from build123d import *

# Parameters (mm, degrees)
SKETCH1_R           = 12.5
BOSS_EXTRUDE1_DEPTH = 75
SKETCH2_R           = 15
BOSS_EXTRUDE2_DEPTH = 20
FILLET1_R           = 2


# Read off the part's stored shape, not the designer's step: Shell2
with BuildPart() as part:
    # Sketch1 → Boss-Extrude1 (new, symmetric)
    with BuildSketch(Plane(origin=(0, 0, 0), x_dir=(1, 0, 0), z_dir=(0, 1, 0))):
        with Locations(Location((0, 0, 0), (0, 0, 270))):
            Circle(SKETCH1_R)
    extrude(amount=BOSS_EXTRUDE1_DEPTH, both=True)

    # Sketch2 → Boss-Extrude2 (add)
    with BuildSketch(Plane(origin=(0, 75, 0), x_dir=(1, 0, 0), z_dir=(0, 1, 0))):
        with Locations(Location((0, 0, 0), (0, 0, 270))):
            Circle(SKETCH2_R)
    boss_extrude2 = extrude(amount=-BOSS_EXTRUDE2_DEPTH)

    # Mirror1: Boss-Extrude2 across plane
    add(boss_extrude2.mirror(Plane.ZX))

    # Fillet1
    fillet1_edges = [part.edges().sort_by_distance(p)[0] for p in [
        (0, -75, -15),
        (0, 75, -15),
    ]]
    fillet(fillet1_edges, radius=FILLET1_R)

    # Shell2 outline → Shell2 (revolve, cut)
    with BuildSketch(Plane.XY):
        with BuildLine():
            Line((13, 74), (0, 74))
            Line((0, 74), (0, -74))
            Line((0, -74), (13, -74))
            ThreePointArc((13, -74), (13.707106781, -73.707106781), (14, -73))
            Line((14, -73), (14, -56))
            Line((14, -56), (11.5, -56))
            Line((11.5, -56), (11.5, 56))
            Line((11.5, 56), (14, 56))
            Line((14, 56), (14, 73))
            ThreePointArc((14, 73), (13.707106781, 73.707106781), (13, 74))
        make_face()
    revolve(axis=Axis((0, 0, 0), (0, 1, 0)), mode=Mode.SUBTRACT)


solid = part.part
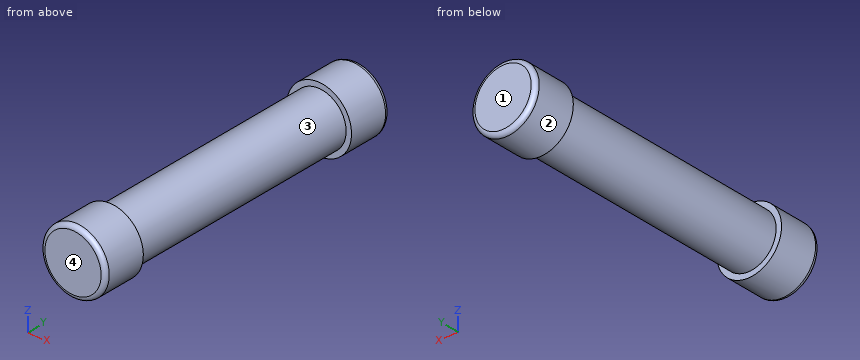
The model under review builds one solid part; all positions refer to its coordinate system, in mm. Face numbers are marked on the shaded views. Round coordinates to 2 decimals unless told otherwise and drop trailing zeros. Order: outer loops, then holes, each group sorted by start corner. A loop starts at its lowest first (then second) coordinate and runs counter-clockwise, first axis right, second up. Notation, with made-up numbers: (19.5, 53) -> (34.5, 53) arc R28 cw to (34.5, 91) -> close; hole circle Ø9 at (69, -0.75). An arc over 180 degrees is marked (long way). Write item = value, one per line. Start each with the question number.
Item 1: For line 1 along Y through (x, z) = (-9.25, 4.75); line 2 along X through (y, z) = (-57.5, 0.75); line 3 along Z through (x, y) = (2.25, 65.5), list the stretches that pass through material, from the lowest coordinate up.
Item 2: Mouldability with a two-part tool opening along Y and no side actions: class the marked faces 1, 2, 3 and 4 as released by +Y, released by -Y, zero draft, split by the parting line, or undercut.
Item 3: Clearance check with flat-ended pins moving along their axes: pin 1 Ø5 at (y, z) = (-30, -10.5) entering from +X; pin 2 Ø1.5 at (y, z) = (32, -11.5) entering from +X; pin 3 Ø5 at (y, z) = (-39.5, 8.5) entering from +X. State where each tip first meets the part, or that it passes through.
Item 4: Consider section A-A on y = -10.5. Write out the cut boundary in (x, z), plus the area to 3 significant figures.
Conclusion:
q1.line_1 = -75 to -74, 74 to 75
q1.line_2 = -14.98 to -13.98, 13.98 to 14.98
q1.line_3 = -14.83 to -13.82, 13.82 to 14.83
q2.face_1 = released by +Y
q2.face_2 = zero draft
q2.face_3 = undercut
q2.face_4 = released by -Y
q3.pin_1 = 9.6
q3.pin_2 = 6.38
q3.pin_3 = 10.97
q4.outline = circle Ø25 at (0, 0); hole circle Ø23 at (0, 0)
q4.area = 75.4 mm2
